Build history of the part. All positions in model axes, mm. Round coordinates to 2 decimals unless told otherwise and drop trailing zeros. Loops run counter-clockwise (first coordinate to the right, second up) from the corner with the lowest first, then second, coordinate; pieces in that order, holes last. Notation, with made-up numbers: (14.5, 68.5) -> (54.5, 68.5) arc R31 ccw to (54.5, 104.5) -> close; hole circle Ø2 at (-14.75, -3). An arc over 180 degrees is marked (long way). Put each result on its own line as item: value. Start each with the question number.
Item 1: Flat gauge pins, fed straight in: pin 1 Ø5 at (x, z) = (-5.5, -10.5) entering from -Y; pin 2 Ø4 at (y, z) = (-2, -18.5) entering from +X; pin 3 Ø2 at (x, y) = (0.5, 6) entering from +Z; pin 4 Ø6 at (x, z) = (-4.5, -8.5) entering from -Y. Where does each tip first touch, or does it go through?
Item 2: Cut at A-A, the plane y = 0. List the corners of the cut face in (x, z).
Item 3: Cut at C-C, the plane z = 19.5. List the corners of the cut face in (x, y), plus the area to 3 significant figures.
Item 4: Drill centre lines: probe 1 along Z at (x, y) = (-6, -4); probe 2 along Y at (x, z) = (-0.25, 13.5); probe 3 along Z at (x, y) = (-4.75, -3). Where is each one in solid material? Low to high. Write a range as [from, to].
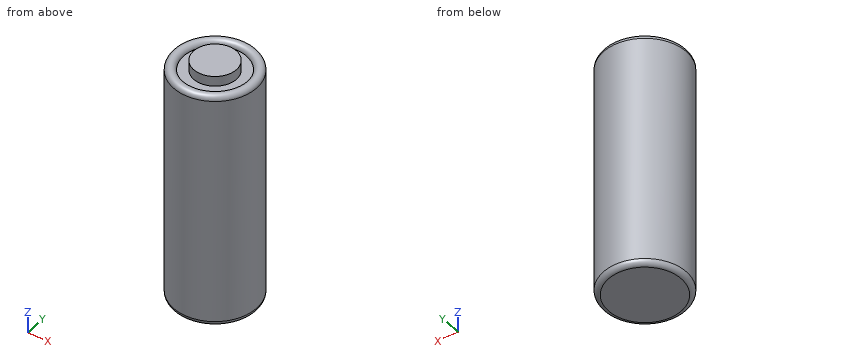
Autodesk Inventor part; units mm, degrees
ref_plane "YZ Plane" through (0, 0, 0) normal (1, 0, 0) x (0, 1, 0)
ref_plane "XZ Plane" through (0, 0, 0) normal (0, 1, 0) x (-1, 0, 0)
ref_plane "XY Plane" through (0, 0, 0) normal (0, 0, 1) x (1, 0, 0)
sketch "Sketch1" plane through (0, 0, 0) normal (0, 0, 1) x (1, 0, 0)
  circle A0 centre (0, 0) radius 8.25
  dimension "d0" = 16.5
extrude "cylinder" add sketch "Sketch1" along normal mid plane 48.5
sketch "Sketch7" plane through (0, 0, 24.25) normal (0, 0, 1) x (1, 0, 0)
  circle A0 centre (0, 0) radius 8.25
  circle A1 centre (0, 0) radius 4.25
  circle A2 centre (0, 0) radius 8.25
  dimension "d17" = 8.5
extrude "button" cut sketch "Sketch7" against normal blind 2
fillet "Fillet1" radius 1 1 edges at (-8.25, 0, -24.25)
sketch "Sketch8" plane through (0, 0, 0) normal (0, 1, 0) x (-1, 0, 0)
  arc A0 (-6.25, 22.25) -> (-8.25, 22.25) centre (-7.25, 22.25) ccw
  line L0 (-8.25, 22.25) -> (8.25, 22.25)
  line L1 (-6.25, 23.25) -> (-8.25, 23.25)
  line L2 (0, -34.65) -> (0, 34.65)
  point P0 (0, 0)
  dimension "d20" = 1
  dimension "d21" = 8.25
revolve "rolled_edge" add sketch "Sketch8" angle 360 about axis through (0, 0, 0) along (0, 0, 1)
properties part number "battery_A_SanyoKR1700AU" material "NiCad"
Reply:
1. pin 1: stops at y = -7.69
1. pin 2: stops at x = 8.25
1. pin 3: stops at z = 23.22
1. pin 4: stops at y = -8.11
2. outline: (-8.25, -23.25) arc R1 ccw to (-7.25, -24.25) -> (7.25, -24.25) arc R1 ccw to (8.25, -23.25) -> (8.25, 22.25) arc R1 ccw to (6.25, 22.25) -> (4.25, 22.25) -> (4.25, 24.25) -> (-4.25, 24.25) -> (-4.25, 22.25) -> (-6.25, 22.25) arc R1 ccw to (-8.25, 22.25) -> close
3. outline: circle Ø16.5 at (0, 0)
3. area: 214 mm^2
4. probe 1: z = [-24.25, 23.25]
4. probe 2: y = [-8.25, 8.25]
4. probe 3: z = [-24.25, 22.25]
